Geometry check sheet. Reference: the model listing, model coordinates, mm. Face numbers are marked on the shaded views. A direction names the side the tool comes from. Coordinates: 2 decimals unless noted, no trailing zeros. Loops run counter-clockwise (first coordinate to the right, second up) from the corner with the lowest first, then second, coordinate; pieces in that order, holes last.
from build123d import *

# Parameters (mm, degrees)
F0_W     = 60
F0_H     = 60
F1_DEPTH = 200
F2_T     = -6
F3_R     = 10
F5_DEPTH = 60.001


with BuildPart() as f1:
    # F0 (on Front) → F1 (new body)
    with BuildSketch(Plane.XZ):
        with Locations((30, 30)):
            Rectangle(F0_W, F0_H)
    extrude(amount=F1_DEPTH)

    # F2
    f2_openings = [f1.faces().sort_by_distance(p)[0] for p in [
        (30, -200, 30),
        (30, 0, 30),
    ]]
    offset(amount=F2_T, openings=f2_openings)

    # F3
    f3_edges = [f1.edges().sort_by_distance(p)[0] for p in [
        (60, -100, 60),
        (0, -100, 60),
        (60, -100, 0),
        (6, -100, 6),
        (0, -100, 0),
        (54, -100, 6),
        (54, -100, 54),
        (6, -100, 54),
    ]]
    fillet(f3_edges, radius=F3_R)

    # F4 (on face) → F5 (cut, through all)
    with BuildSketch(Plane.XY.offset(60)):
        Polygon((0, 0), (70, -40.4145188433), (70, 0), align=None)
    extrude(amount=-F5_DEPTH, mode=Mode.SUBTRACT)


solid = f1.part
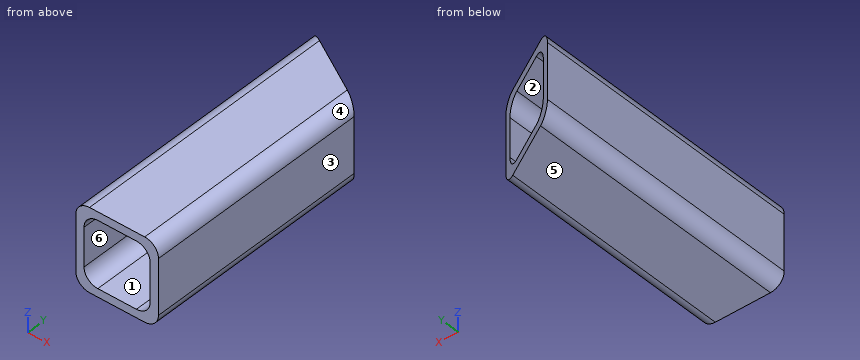
(1) Scan lines: L1, parallel to Z at x = 27.5, y = -94; L2, parallel to X at y = -126, z = 44.5; L3, parallel to Y at x = 54, z = 3. Record each from-to range of solid material in increasing order.
Findings:
L1: z = 0 to 6, 54 to 60
L2: x = 0 to 6.01, 53.99 to 60
L3: y = -200 to -31.18
(2) Sectioned sample at C-C on z = 25.5. Record the cut outline in (x, y).
Findings:
outline: (0, -200) - (6, -200) - (6, -3.46) - (0, 0) - close; (54, -200) - (60, -200) - (60, -34.64) - (54, -31.18) - close
(3) Sectioned sample at A-A on y = -157. Record the cut outline in (x, z), and give its area (3 significant figures).
Findings:
outline: (0, 10) arc R10 ccw to (10, 0) - (50, 0) arc R10 ccw to (60, 10) - (60, 50) arc R10 ccw to (50, 60) - (10, 60) arc R10 ccw to (0, 50) - close; hole (6, 16) arc R10 ccw to (16, 6) - (44, 6) arc R10 ccw to (54, 16) - (54, 44) arc R10 ccw to (44, 54) - (16, 54) arc R10 ccw to (6, 44) - close
area: 1,300 mm2
(4) Sectioned sample at B-B on x = 29. Record the cut outline in (y, z), and give its area (3 significant figures).
Findings:
outline: (-200, 0) - (-16.74, 0) - (-16.74, 6) - (-200, 6) - close; (-200, 54) - (-16.74, 54) - (-16.74, 60) - (-200, 60) - close
area: 2,200 mm2
(5) Access from +Z, -Z, +X, -X, +Y, -Y to the whole of each face (thin tool, end or side, straight path). Record for the marked faces 5 and 6.
Findings:
face 5: -Z, +X, -X, +Y, -Y
face 6: +Y, -Y
(6) Sectioned sample at D-D on y = -14. Record the cut outline in (x, z).
Findings:
outline: (0, 10) arc R10 ccw to (10, 0) - (24.25, 0) - (24.25, 6) - (16, 6) arc R10 cw to (6, 16) - (6, 44) arc R10 cw to (16, 54) - (24.25, 54) - (24.25, 60) - (10, 60) arc R10 ccw to (0, 50) - close
(7) Draft check along Z on the marked faces 1, 2, 3 and 4. Enter one of: +Z half, -Z half, draft (parallel to the pull), parting line (faces both ways), or undercut.
Findings:
face 1: undercut
face 2: undercut
face 3: draft
face 4: +Z half
(8) Gauge pin test, flat end, axial feed: pin 1 Ø5 at (x, y) = (7, -60.5) entering from -Z. Record the tip position at first contact, or that the pin passes through.
Findings:
pin 1: stops at z = 0.01
